from build123d import *

# Parameters (mm, degrees)
SKETCH1_R           = 1.5
EXTRUDE1_DEPTH      = 5
EXTRUDE1_DEPTH_BACK = 5


with BuildPart() as part:
    # Sketch1 → Extrude1 (new body, two sides)
    with BuildSketch(Plane.XY) as extrude1_sk:
        Polygon((0, 2.598076211), (-2.25, 1.299038106), (-2.25, -1.299038106), (0, -2.598076211), (2.25, -1.299038106), (2.25, 1.299038106), align=None)
        Circle(SKETCH1_R, mode=Mode.SUBTRACT)
    extrude(amount=EXTRUDE1_DEPTH)
    extrude(extrude1_sk.sketch, amount=-EXTRUDE1_DEPTH_BACK)


solid = part.part
CAD build for the part. Positions are in the model's coordinates, mm. Round coordinates to 2 decimals unless told otherwise and drop trailing zeros. Write each loop counter-clockwise with the first axis right and the second up, starting at its lowest first coordinate (ties: lowest second). Pieces come first, ordered by that corner, then holes. Notation, with made-up numbers: M 84.25,-8.5 L 111.25,-8.5 A9 cw 111.25,8.5 Z; hole C -4.5,72 d8. An arc over 180 degrees is marked long. Use a Markdown table: item, result. Add a question column.
1. Slice it at B-B on x = 1.4. Give the cut face in (y, z), then the cut area to 3 significant figures.
2. Slice it at C-C on y = 0. Give the cut face in (x, z), then the cut area to 3 significant figures.
3. Drill centre lines: probe 1 along Y at (x, z) = (0.65, 0); probe 2 along Y at (x, z) = (0.8, 0.5); probe 3 along X at (y, z) = (-1.1, 2). Where is each one in solid material? Low to high.
4. Pull direction X, two halves, no side cores. Call faces 1 (the face through (2.25, 0, 0)), 2 (the face through (-1.5, 0.07, -0.07)), 3 (the face through (-1.109, 1.958, 0.07)): released by +X, released by -X, zero draft, split by the parting line, or undercut.
5. Slice it at A-A on z = 1.5. Give the cut face in (x, y), then the cut area to 3 significant figures.
6. Slice it at D-D on y = 1.65. Give the cut face in (x, z), then the cut area to 3 significant figures.
7. Flat gauge pin, fed straight in: P1, Ø1.5, axis at x = -1, z = 0.5, coming from the -Y side. Where does the tip first touch, or does it go through?
Reply:
| question | item | result |
|---|---|---|
| 1 | outline | M -1.79,-5 L -0.54,-5 L -0.54,5 L -1.79,5 Z; M 0.54,-5 L 1.79,-5 L 1.79,5 L 0.54,5 Z |
| 1 | area | 25.0 mm^2 |
| 2 | outline | M -2.25,-5 L -1.5,-5 L -1.5,5 L -2.25,5 Z; M 1.5,-5 L 2.25,-5 L 2.25,5 L 1.5,5 Z |
| 2 | area | 15.0 mm^2 |
| 3 | probe 1 | y = -2.22 to -1.35, 1.35 to 2.22 |
| 3 | probe 2 | y = -2.14 to -1.27, 1.27 to 2.14 |
| 3 | probe 3 | x = -2.25 to -1.02, 1.02 to 2.25 |
| 4 | face 1 | released by +X |
| 4 | face 2 | undercut |
| 4 | face 3 | released by -X |
| 5 | outline | M -2.25,-1.3 L 0,-2.6 L 2.25,-1.3 L 2.25,1.3 L 0,2.6 L -2.25,1.3 Z; hole C 0,0 d3 |
| 5 | area | 10.5 mm^2 |
| 6 | outline | M -1.64,-5 L 1.64,-5 L 1.64,5 L -1.64,5 Z |
| 6 | area | 32.8 mm^2 |
| 7 | P1 | stops at y = -2.45 |
